from build123d import *

# Parameters (mm, degrees)
F0_W     = 25.4
F0_H     = 25.4
F1_DEPTH = 6.35
F3_DEPTH = 25.4
F4_R     = 1.3225172329
F5_DEPTH = 25.4


# Not quite as in the source:
# - a feature names something its author has since deleted; it is built from what else it names


with BuildPart() as f1:
    # F0 (on Front) → F1 (new body)
    with BuildSketch(Plane.XZ):
        with Locations((12.7, 12.7)):
            Rectangle(F0_W, F0_H)
    extrude(amount=F1_DEPTH)

    # F2 (on face) → F3 (cut)
    with BuildSketch(Plane.XZ.offset(6.35)):
        with BuildLine():
            ThreePointArc((4.347079063, 12.7), (5.4149768535, 6.5815794315), (10.3514468814, 2.8123965482))
            Line((10.3514468814, 2.8123965482), (10.3514468814, 21.082))
            ThreePointArc((10.3514468814, 21.082), (10.2026571262, 21.4412102448), (9.8434468814, 21.59))
            Line((9.8434468814, 21.59), (5.08, 21.59))
            ThreePointArc((5.08, 21.59), (4.3615795103, 21.8875795103), (4.064, 22.606))
            Line((4.064, 22.606), (4.064, 24.384))
            ThreePointArc((4.064, 24.384), (4.3615795103, 25.1024204897), (5.08, 25.4))
            Line((5.08, 25.4), (0, 25.4))
            Line((0, 25.4), (0, 0))
            Line((0, 0), (11.9920649295, 0))
            ThreePointArc((11.9920649295, 0), (3.957639074, 4.0680963279), (1.3902190546, 12.7))
            ThreePointArc((1.3902190546, 12.7), (0.7220113765, 13.0957453087), (0.7478720811, 13.8719199503))
            Line((0.7478720811, 13.8719199503), (2.1310466878, 16.0393626953))
            ThreePointArc((2.1310466878, 16.0393626953), (2.7505395089, 16.3910999432), (3.390007158, 16.0771388424))
            Line((3.390007158, 16.0771388424), (4.9636925598, 13.9096960974))
            ThreePointArc((4.9636925598, 13.9096960974), (5.025970964, 13.1159511785), (4.347079063, 12.7))
        make_face()
        with BuildLine():
            Line((25.4, 25.4), (20.32, 25.4))
            ThreePointArc((20.32, 25.4), (21.0384204897, 25.1024204897), (21.336, 24.384))
            Line((21.336, 24.384), (21.336, 22.606))
            ThreePointArc((21.336, 22.606), (21.0384204897, 21.8875795103), (20.32, 21.59))
            Line((20.32, 21.59), (15.5565531186, 21.59))
            ThreePointArc((15.5565531186, 21.59), (15.1973428738, 21.4412102448), (15.0485531186, 21.082))
            Line((15.0485531186, 21.082), (15.0485531186, 15.5096852131))
            Line((15.0485531186, 15.5096852131), (15.0485531186, 2.8123965482))
            ThreePointArc((15.0485531186, 2.8123965482), (19.9850231465, 6.5815794315), (21.052920937, 12.7))
            ThreePointArc((21.052920937, 12.7), (20.374029036, 13.1159511785), (20.4363074402, 13.9096960974))
            Line((20.4363074402, 13.9096960974), (22.009992842, 16.0771388424))
            ThreePointArc((22.009992842, 16.0771388424), (22.6494604911, 16.3910999432), (23.2689533122, 16.0393626953))
            Line((23.2689533122, 16.0393626953), (24.6521279189, 13.8719199503))
            ThreePointArc((24.6521279189, 13.8719199503), (24.6779886235, 13.0957453087), (24.0097809454, 12.7))
            ThreePointArc((24.0097809454, 12.7), (21.442360926, 4.0680963279), (13.4079350705, 0))
            Line((13.4079350705, 0), (25.4, 0))
            Line((25.4, 0), (25.4, 25.4))
        make_face()
    extrude(amount=-F3_DEPTH, mode=Mode.SUBTRACT)

    # F4 (on Front) → F5 (cut)
    with BuildSketch(Plane.XZ):
        with Locations((12.7565525472, 23.5501565039)):
            Circle(F4_R)
    extrude(amount=F5_DEPTH, mode=Mode.SUBTRACT)


solid = f1.part
Here's how the part is built. I have some questions about the finished solid (model axes, mm). A direction names the side the tool comes from. Round coordinates to 2 decimals unless told otherwise and drop trailing zeros. Order: outer loops, then holes, each group sorted by start corner. A loop starts at its lowest first (then second) coordinate and runs counter-clockwise, first axis right, second up. Notation, with made-up numbers: (18, -7.5) -> (45, -7.5) arc R12 cw to (45, -3.5) -> close; hole circle Ø4 at (20, 89). An arc over 180 degrees is marked (long way). Return JSON: item names as keys, results as strings.
Q1. For pin 1 Ø2 at (y, z) = (-4.5, 23.5) entering from -X; pin 2 Ø1.9 at (y, z) = (-3.5, 12) entering from -X; pin 3 Ø0.5 at (y, z) = (-2.5, 23.5) entering from +X, each with a flat end and sliding along its axis, tell me the tip position at first contact or that it passes through.
Filled sheet:
{"pin 1": "stops at x = 4.06", "pin 2": "stops at x = 0.83", "pin 3": "stops at x = 21.34"}
Q2. If we mould it in two halves opening along Z, with no side actions, what happens to faces 1 (the cylindrical face through (2.74, -3.22, 16.39)), 2 (the flat face through (13, -6.35, 13)), 3 (the cylindrical face through (14, -3, 24))? For each: released by +Z, released by -Z, zero draft, split by the parting line, or undercut.
Filled sheet:
{"face 1": "released by +Z", "face 2": "zero draft", "face 3": "undercut"}
Q3. If we section it at A-A on x = 19.5: List the corners of the cut face in (y, z) for me.
Filled sheet:
{"outline": "(-6.35, 2.23) -> (0, 2.23) -> (0, 5.87) -> (-6.35, 5.87) -> close; (-6.35, 21.59) -> (0, 21.59) -> (0, 25.4) -> (-6.35, 25.4) -> close"}
Q4. If we section it at C-C on z = 2: List the corners of the cut face in (x, y) for me.
Filled sheet:
{"outline": "(6.22, -6.35) -> (19.18, -6.35) -> (19.18, 0) -> (6.22, 0) -> close"}
Q5. Which directions (+Z, -Z, +X, -X, +Y, -Y) give clear straight access to the entire face, cutting with the end or side of a thin tool? Please do faces 4 (the cylindrical face through (21.03, -3.22, 25.11)), 5 (the flat face through (4.166, -3.219, 15.009)), 6 (the flat face through (4.064, -3, 23)), 7 (the flat face through (18, -3, 21.59)), 8 (the flat face through (7, -3, 21.59)).
Filled sheet:
{"face 4": "+Z, +X, +Y, -Y", "face 5": "+Y, -Y", "face 6": "+Z, -X, +Y, -Y", "face 7": "+X, +Y, -Y", "face 8": "-X, +Y, -Y"}
Q6. I need wall thicknesses on line 1 along X through (y, z) = (-0.25, 13.5); line 2 along X through (y, z) = (-0.5, 15); line 3 along Z through (x, y) = (20, -4). Which ranges of each line are inside material? Lowest first, please. Write a range as from..to.
Filled sheet:
{"line 1": "x = 0.63..5.11, 10.35..15.05, 20.29..24.77", "line 2": "x = 1.47..4.17, 10.35..15.05, 21.23..23.93", "line 3": "z = 2.63..6.61, 21.59..25.4"}
